Here's the drawing with two shaded views (mm, measured from the low corner). I have some questions. A direction names the side the tool comes from. Coordinates: 2 decimals unless noted, no trailing zeros. Write each loop counter-clockwise with the first axis right and the second up, starting at its lowest first coordinate (ties: lowest second). Pieces come first, ordered by that corner, then holes. Notation, with made-up numbers: (72, 86) -> (89, 86) arc R25 cw to (89, 108) -> close; hole circle Ø10 at (-5.75, 20). An arc over 180 degrees is marked (long way). Put each result on its own line as item: value.
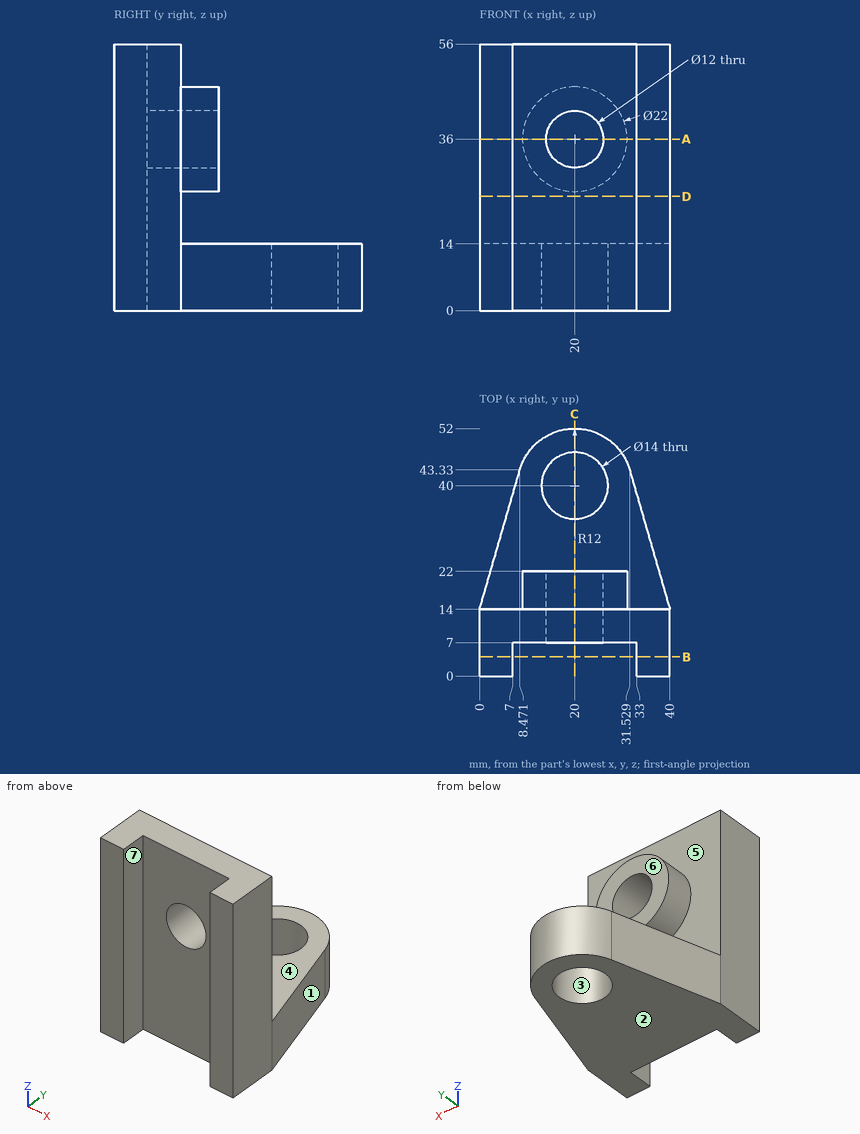
Item 1: Imagine slicing it at D-D on z = 24. Write out the boundary of the cut face in (x, y), then the cut area to 3 significant figures.
Output:
outline: (0, 0) -> (7, 0) -> (7, 7) -> (33, 7) -> (33, 0) -> (40, 0) -> (40, 14) -> (0, 14) -> close
area: 378 mm²
Item 2: Imagine slicing it at B-B on y = 4. Write out the boundary of the cut face in (x, z), then the cut area to 3 significant figures.
Output:
outline: (0, 0) -> (7, 0) -> (7, 56) -> (0, 56) -> close; (33, 0) -> (40, 0) -> (40, 56) -> (33, 56) -> close
area: 784 mm²
Item 3: Please list where these lines run through material, in increasing order: line 1 along X through (y, z) = (2, 31.5); line 2 along X through (y, z) = (17.75, 36); line 3 along Y through (x, z) = (20, 9.25). Write a range as from..to.
Output:
line 1: x = 0..7, 33..40
line 2: x = 9..14, 26..31
line 3: y = 7..33, 47..52
Item 4: For P1, Ø2, axis at y = 42, z = 5.5, coming from the -X side; P2, Ø12, axis at x = 16, z = 17, coming from the -Y side; P3, Ø11, axis at x = 20, y = 40, coming from the -Z side; P4, Ø8, axis at x = 7, z = 29, coming from the +Y side, each with a flat end and sliding along its axis, tell me the tip position at first contact or that it passes through.
Output:
P1: stops at x = 7.8
P2: stops at y = 7
P3: passes through
P4: stops at y = 22
Item 5: Imagine slicing it at C-C on x = 20. Write out the boundary of the cut face in (y, z).
Output:
outline: (7, 0) -> (33, 0) -> (33, 14) -> (14, 14) -> (14, 25) -> (22, 25) -> (22, 30) -> (7, 30) -> close; (7, 42) -> (22, 42) -> (22, 47) -> (14, 47) -> (14, 56) -> (7, 56) -> close; (47, 0) -> (52, 0) -> (52, 14) -> (47, 14) -> close
Item 6: Imagine slicing it at A-A on z = 36. Write out the boundary of the cut face in (x, y), then the cut area to 3 significant figures.
Output:
outline: (0, 0) -> (7, 0) -> (7, 7) -> (14, 7) -> (14, 22) -> (9, 22) -> (9, 14) -> (0, 14) -> close; (26, 7) -> (33, 7) -> (33, 0) -> (40, 0) -> (40, 14) -> (31, 14) -> (31, 22) -> (26, 22) -> close
area: 374 mm²
Item 7: Which directions (+Z, -Z, +X, -X, +Y, -Y) give clear straight access to the entire face, cutting with the end or side of a thin tool? Please do the marked faces 4, 5, 6 and 7.
Output:
face 4: +X, -X, +Y
face 5: +Y
face 6: +Z, +X, -X, +Y
face 7: +Z, -Z, -Y
Item 8: If we mould it in two halves opening along X, with no side actions, what happens to the marked faces 1, 2 and 3? For each: released by +X, released by -X, zero draft, split by the parting line, or undercut.
Output:
face 1: released by +X
face 2: zero draft
face 3: undercut
